Can you work these out from the model? Positions are in its coordinate system, mm. Face numbers are marked on the shaded views. Give positions to 0.01 mm unless a question says otherwise; leave off trailing zeros. Order: outer loops, then holes, each group sorted by start corner. A loop starts at its lowest first (then second) coordinate and runs counter-clockwise, first axis right, second up. Notation, with made-up numbers: (4.25, -22) - (54.25, -22) arc R20 ccw to (54.25, -9) - close; hole circle Ø6 at (-35.5, 44.5). An arc over 180 degrees is marked (long way). Use one line per item in the form item = value. Start each with the question number.
1) We'd pull the mould along Y, two halves only. Please class the marked faces 1, 2, 3 and 4: released by +Y, released by -Y, zero draft, split by the parting line, or undercut.
2) Suppose I cut it at D-D, the plane x = 29.5. Write out the boundary of the cut face in (y, z).
3) For pin 1 (1 mm diameter, centred on x = 23.5, z = -3.5, fed in from +Y) (3 decimals), with a flat end and sliding along its axis, tell me the tip position at first contact or that it passes through.
4) Please list where these lines run through material, in increasing order: probe 1 along X at (y, z) = (7.25, -4); probe 2 along X at (y, z) = (1.25, -4.75); probe 3 along Y at (x, z) = (52, -0.5) (3 decimals).
5) Suppose I cut it at A-A, the plane y = 1.75. Write out the boundary of the cut face in (x, z), and give its area (3 significant figures).
6) Suppose I cut it at B-B, the plane y = 4.5. Write out the boundary of the cut face in (x, z).
7) Suppose I cut it at C-C, the plane x = 15.5. Write out the boundary of the cut face in (y, z), and give its area (3 significant figures).
```python
from build123d import *

# Parameters (mm, degrees)
BLANKSKE_W        = 61
BLANKSKE_H        = 14.5
BLANK_DEPTH       = 6.5
TOOTHCUTSIM_DEPTH = 64.035704168
TEETHCUTS_COUNT   = 14
TEETHCUTS_PITCH   = 4.712388975
DOVETAIL_DEPTH    = 6.5


with BuildPart() as part:
    # BlankSke → Blank (new body)
    with BuildSketch(Plane.XY):
        with Locations((30.5, 7.25)):
            Rectangle(BLANKSKE_W, BLANKSKE_H)
    extrude(amount=-BLANK_DEPTH)

    # TooCutSkeSim → ToothCutSim (cut, through all)
    with BuildSketch(Plane.XY):
        Polygon((0.654653055, 11.125), (-0.654653055, 11.125), (-1.892297439, 14.5254), (1.892297439, 14.5254), align=None)
    toothcutsim = extrude(amount=-TOOTHCUTSIM_DEPTH, mode=Mode.SUBTRACT)

    # TeethCuts: ToothCutSim ×14
    with Locations(*[(i * TEETHCUTS_PITCH, 0, 0) for i in range(1, TEETHCUTS_COUNT)]):
        add(toothcutsim, mode=Mode.SUBTRACT)

    # Sketch2 → Dovetail (cut)
    with BuildSketch(Plane.XY):
        with BuildLine():
            Line((13, 8.625), (4, 8.625))
            ThreePointArc((4, 8.625), (2.673189596, 7.824695756), (2.762181855, 6.277765535))
            Line((2.762181855, 6.277765535), (5.126060485, 2.824114884))
            ThreePointArc((5.126060485, 2.824114884), (5.776520827, 1.478123401), (6, 0))
            Line((6, 0), (11, 0))
            ThreePointArc((11, 0), (11.223479173, 1.478123401), (11.873939515, 2.824114884))
            Line((11.873939515, 2.824114884), (14.237818145, 6.277765535))
            ThreePointArc((14.237818145, 6.277765535), (14.326810404, 7.824695756), (13, 8.625))
        make_face()
    extrude(amount=-DOVETAIL_DEPTH, mode=Mode.SUBTRACT)


solid = part.part
```
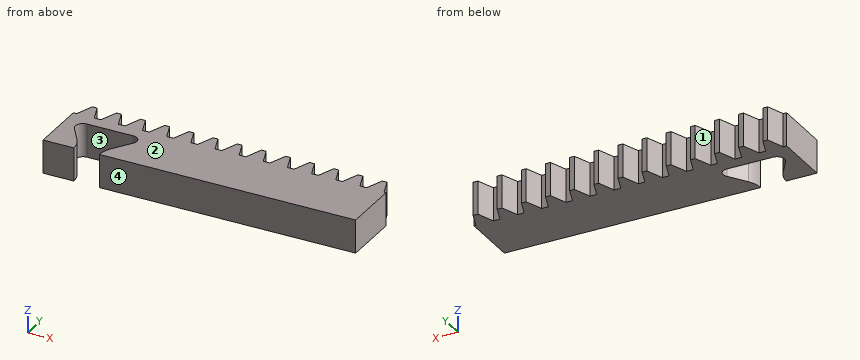
Result sheet:
q1.face_1 = released by +Y
q1.face_2 = zero draft
q1.face_3 = undercut
q1.face_4 = released by -Y
q2.outline = (0, -6.5) - (12.69, -6.5) - (12.69, 0) - (0, 0) - close
q3.pin_1 = 11.125
q4.probe_1 = 0 to 2.51, 14.49 to 61
q4.probe_2 = 0 to 5.84, 11.16 to 61
q4.probe_3 = 0 to 11.125
q5.outline = (0, -6.5) - (5.68, -6.5) - (5.68, 0) - (0, 0) - close; (11.32, -6.5) - (61, -6.5) - (61, 0) - (11.32, 0) - close
q5.area = 360 mm²
q6.outline = (0, -6.5) - (3.98, -6.5) - (3.98, 0) - (0, 0) - close; (13.02, -6.5) - (61, -6.5) - (61, 0) - (13.02, 0) - close
q7.outline = (0, -6.5) - (13.07, -6.5) - (13.07, 0) - (0, 0) - close
q7.area = 85.0 mm²
